For this review, take the finished solid that the model builds, in its own axes (mm). A direction names the side the tool comes from. Give positions to 0.01 mm unless a question says otherwise; leave off trailing zeros. Write each loop counter-clockwise with the first axis right and the second up, starting at its lowest first coordinate (ties: lowest second). Pieces come first, ordered by that corner, then holes. Notation, with made-up numbers: (21.5, 17.25) -> (48.5, 17.25) arc R14 cw to (48.5, 22.25) -> close; hole circle Ø6 at (16, 53). An arc over 180 degrees is marked (long way). Answer as CSV lines item,"result".
```python
from build123d import *

# Parameters (mm, degrees)
SKETCH1_R           = 3
BOSS_EXTRUDE1_DEPTH = 3
SKETCH2_R           = 1.5
BOSS_EXTRUDE2_DEPTH = 25
CHAMFER1_SIZE       = 0.2
CUT_EXTRUDE1_DEPTH  = 2


with BuildPart() as part:
    # Sketch1 → Boss-Extrude1 (new body)
    with BuildSketch(Plane(origin=(0, 0, 0), x_dir=(1, 0, 0), z_dir=(0, 1, 0))):
        with Locations(Location((0, 0, 0), (0, 0, 270))):
            Circle(SKETCH1_R)
    extrude(amount=BOSS_EXTRUDE1_DEPTH)

    # Sketch2 → Boss-Extrude2 (add)
    with BuildSketch(Plane(origin=(0, 3, 0), x_dir=(1, 0, 0), z_dir=(0, 1, 0))):
        with Locations(Location((0, 0, 0), (0, 0, 270))):
            Circle(SKETCH2_R)
    extrude(amount=BOSS_EXTRUDE2_DEPTH)

    # Chamfer1
    chamfer1_edges = [part.edges().sort_by_distance(p)[0] for p in [
        (0, 28, -1.5),
    ]]
    chamfer(chamfer1_edges, length=CHAMFER1_SIZE)

    # Sketch3 → Cut-Extrude1 (cut)
    with BuildSketch(Plane.XZ):
        Polygon((0, 1.529103694), (-1.324242644, 0.764551847), (-1.324242644, -0.764551847), (0, -1.529103694), (1.324242644, -0.764551847), (1.324242644, 0.764551847), align=None)
    extrude(amount=-CUT_EXTRUDE1_DEPTH, mode=Mode.SUBTRACT)


solid = part.part
```
Q1. Draft analysis for pull direction Z (two halves, no side actions). For faces 1 (the cylindrical face through (0.9, 1.48, 2.86)), 2 (the flat face through (1.324, 1, 0)), 3 (the flat face through (0.7, 0, 1.3)), state which applies: released by +Z, released by -Z, zero draft, split by the parting line, or undercut.
Answer block:
face 1,"split by the parting line"
face 2,"undercut"
face 3,"zero draft"
Q2. For faces 4 (the cylindrical face through (0.45, 15.23, 1.43)), 5 (the flat face through (0.653, 0.986, -1.152)), 6 (the flat face through (0, 28, 0)), list the 3-axis set-ups (+Z, -Z, +X, -X, +Y, -Y) from which the entire face can be reached by the end or side of a thin tool; tool diameter is ignored.
Answer block:
face 4,"+Y"
face 5,"-Y"
face 6,"+Z, -Z, +X, -X, +Y"
Q3. Clearance check with flat-ended pins moving along their axes: pin 1 (1.5 mm diameter, centred on y = 24.5, z = 1.5, fed in from -X); pin 2 (3 mm diameter, centred on y = 11, z = 1.5, fed in from -X). State where each tip first meets the part, or that it passes through.
Answer block:
pin 1,"stops at x = -1.3"
pin 2,"stops at x = -1.5"
Q4. Add section A-A (z = 0). Write out the cut boundary in (x, y).
Answer block:
outline,"(-3, 0) -> (-1.32, 0) -> (-1.32, 2) -> (1.32, 2) -> (1.32, 0) -> (3, 0) -> (3, 3) -> (1.5, 3) -> (1.5, 27.8) -> (1.3, 28) -> (-1.3, 28) -> (-1.5, 27.8) -> (-1.5, 3) -> (-3, 3) -> close"
Q5. Add section D-D (z = -1.8). Write out the cut boundary in (x, y), plus the area to 3 significant figures.
Answer block:
outline,"(-2.4, 0) -> (2.4, 0) -> (2.4, 3) -> (-2.4, 3) -> close"
area,"14.4 mm2"
Q6. To check wall thickness, follow probe 1 along Y at (x, z) = (-2.35, -0.1); probe 2 along Y at (x, z) = (0.45, 1.2); probe 3 along X at (y, z) = (23, 0.05). State the ranges of each line that lie inside material, in increasing order. Write a range as [from, to].
Answer block:
probe 1,"y = [0, 3]"
probe 2,"y = [2, 28]"
probe 3,"x = [-1.5, 1.5]"
Q7. Add section B-B (y = 8.75). Write out the cut boundary in (x, z), plus the area to 3 significant figures.
Answer block:
outline,"circle Ø3 at (0, 0)"
area,"7.07 mm2"
Q8. Add section C-C (x = -1.8). Write out the cut boundary in (y, z), plus the area to 3 significant figures.
Answer block:
outline,"(0, -2.4) -> (3, -2.4) -> (3, 2.4) -> (0, 2.4) -> close"
area,"14.4 mm2"
